The model under review builds one solid part; all positions refer to its coordinate system, in mm. Round coordinates to 2 decimals unless told otherwise and drop trailing zeros. Order: outer loops, then holes, each group sorted by start corner. A loop starts at its lowest first (then second) coordinate and runs counter-clockwise, first axis right, second up.
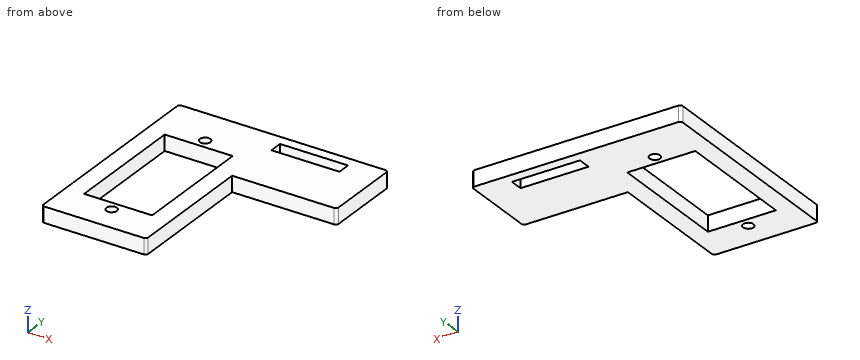
```python
from build123d import *

# Parameters (mm, degrees)
IZIM1_W                     = 13
IZIM1_H                     = 23.5
Y_KSEKLIK_EKSTR_ZYON1_DEPTH = 3
RADYUS1_R                   = 0.5
KES_EKSTR_ZYON1_REACH       = 38.886
IZIM5_R                     = 1
KES_EKSTR_ZYON2_REACH       = 38.886
IZIM6_W                     = 13
IZIM6_H                     = 2.5


with BuildPart() as part:
    # Çizim1 → Yükseklik-Ekstrüzyon1 (new body)
    with BuildSketch(Plane.XY):
        Polygon((10, 21.25), (30, 21.25), (30, 6.25), (10, 6.25), (10, -18.75), (-10, -18.75), (-10, 21.25), align=None)
        Rectangle(IZIM1_W, IZIM1_H, mode=Mode.SUBTRACT)
    extrude(amount=Y_KSEKLIK_EKSTR_ZYON1_DEPTH)

    # Radyus1
    radyus1_edges = [part.edges().sort_by_distance(p)[0] for p in [
        (-10, 21.25, 1.5),
        (30, 21.25, 1.5),
        (30, 6.25, 1.5),
        (10, -18.75, 1.5),
        (-10, -18.75, 1.5),
    ]]
    fillet(radyus1_edges, radius=RADYUS1_R)

    # Çizim5 → Kes-Ekstrüzyon1 (cut, up to next)
    with BuildSketch(Plane(origin=(0, 0, 0), x_dir=(-1, 0, 0), z_dir=(0, 0, -1)), mode=Mode.PRIVATE) as kes_ekstr_zyon1_sk1:
        with Locations((0, 13.625)):
            Circle(IZIM5_R)
    kes_ekstr_zyon1_tool1 = extrude(kes_ekstr_zyon1_sk1.sketch, amount=-KES_EKSTR_ZYON1_REACH, mode=Mode.PRIVATE) & part.part
    # Çizim5 → Kes-Ekstrüzyon1 (cut, up to next)
    with BuildSketch(Plane(origin=(0, 0, 0), x_dir=(-1, 0, 0), z_dir=(0, 0, -1)), mode=Mode.PRIVATE) as kes_ekstr_zyon1_sk2:
        with Locations((0, -13.625)):
            Circle(IZIM5_R)
    kes_ekstr_zyon1_tool2 = extrude(kes_ekstr_zyon1_sk2.sketch, amount=-KES_EKSTR_ZYON1_REACH, mode=Mode.PRIVATE) & part.part
    add(kes_ekstr_zyon1_tool1.solids().sort_by_distance((0, 13.625, 0))[0], mode=Mode.SUBTRACT)
    add(kes_ekstr_zyon1_tool2.solids().sort_by_distance((0, -13.625, 0))[0], mode=Mode.SUBTRACT)

    # Çizim6 → Kes-Ekstrüzyon2 (cut, up to next)
    with BuildSketch(Plane(origin=(0, 0, 0), x_dir=(-1, 0, 0), z_dir=(0, 0, -1)), mode=Mode.PRIVATE) as kes_ekstr_zyon2_sk1:
        with Locations((-17.130228212, 18)):
            Rectangle(IZIM6_W, IZIM6_H)
    kes_ekstr_zyon2_tool1 = extrude(kes_ekstr_zyon2_sk1.sketch, amount=-KES_EKSTR_ZYON2_REACH, mode=Mode.PRIVATE) & part.part
    add(kes_ekstr_zyon2_tool1.solids().sort_by_distance((17.130228, 18, 0))[0], mode=Mode.SUBTRACT)


solid = part.part
```
(1) To check wall thickness, follow probe 1 along Y at (x, z) = (0, 1.25) (3 decimals); probe 2 along X at (y, z) = (0, 0.65); probe 3 along Y at (x, z) = (-3, 1.1). State the ranges of each line that lie inside material, in increasing order.
Data:
probe 1: y = -18.75 to -14.625, -12.625 to -11.75, 11.75 to 12.625, 14.625 to 21.25
probe 2: x = -10 to -6.5, 6.5 to 10
probe 3: y = -18.75 to -11.75, 11.75 to 21.25
(2) Consider section D-D (z = 0.55). Write out the cut boundary in (x, y) (3 decimals).
Data:
outline: (-10, -18.25) arc R0.5 ccw to (-9.5, -18.75) - (9.5, -18.75) arc R0.5 ccw to (10, -18.25) - (10, 6.25) - (29.5, 6.25) arc R0.5 ccw to (30, 6.75) - (30, 20.75) arc R0.5 ccw to (29.5, 21.25) - (-9.5, 21.25) arc R0.5 ccw to (-10, 20.75) - close; hole (-6.5, -11.75) - (6.5, -11.75) - (6.5, 11.75) - (-6.5, 11.75) - close; hole circle Ø2 at (0, -13.625); hole circle Ø2 at (0, 13.625); hole (10.63, 16.75) - (23.63, 16.75) - (23.63, 19.25) - (10.63, 19.25) - close
(3) Insertion check: pin 1 (1.5 mm diameter, centred on y = 3.5, z = 2, fed in from +X); pin 2 (6 mm diameter, centred on x = 7, y = 7.5, fed in from -Z). Each pin has a flat end and moves straight along its axis. Give the tip position at first contact, or say it passes through.
Data:
pin 1: stops at x = 10
pin 2: stops at z = 0
(4) Consider section C-C (x = 0). Write out the cut boundary in (y, z) (3 decimals), and give its area (3 significant figures).
Data:
outline: (-18.75, 0) - (-14.625, 0) - (-14.625, 3) - (-18.75, 3) - close; (-12.625, 0) - (-11.75, 0) - (-11.75, 3) - (-12.625, 3) - close; (11.75, 0) - (12.625, 0) - (12.625, 3) - (11.75, 3) - close; (14.625, 0) - (21.25, 0) - (21.25, 3) - (14.625, 3) - close
area: 37.5 mm2
(5) Consider section B-B (y = 2.5). Write out the cut boundary in (x, z), and give its area (3 significant figures).
Data:
outline: (-10, 0) - (-6.5, 0) - (-6.5, 3) - (-10, 3) - close; (6.5, 0) - (10, 0) - (10, 3) - (6.5, 3) - close
area: 21.0 mm2
(6) Consider section A-A (x = 5). Write out the cut boundary in (y, z).
Data:
outline: (-18.75, 0) - (-11.75, 0) - (-11.75, 3) - (-18.75, 3) - close; (11.75, 0) - (21.25, 0) - (21.25, 3) - (11.75, 3) - close
